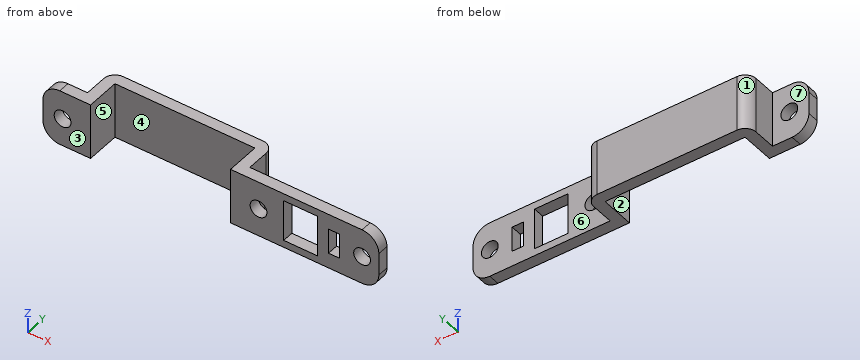
from build123d import *

# Parameters (mm, degrees)
EXTRUIR_L_MINA1_DEPTH = 10
CROQUIS2_R            = 1.5
CORTAR_EXTRUIR1_DEPTH = 61.141499815
REDONDEO2_R           = 3
REDONDEO3_R           = 2
CROQUIS3_W            = 6
CROQUIS3_H            = 7.4
CROQUIS3_W_2          = 2
CROQUIS3_H_2          = 4.5
CORTAR_EXTRUIR2_DEPTH = 61.141499815


with BuildPart() as part:
    # Croquis1 → Extruir-Lámina1 (new body)
    with BuildSketch(Plane.XY):
        Polygon((-1, 0), (0, 0), (7.5, 0), (7.5, 6), (32.5, 6), (32.5, 0), (41.5, 0), (59, 0), (59, 2), (41.5, 2), (34.5, 2), (34.5, 8), (5.5, 8), (5.5, 2), (0, 2), (-1, 2), align=None)
    extrude(amount=-EXTRUIR_L_MINA1_DEPTH)

    # Croquis2 → Cortar-Extruir1 (cut, through all)
    with BuildSketch(Plane(origin=(0, 2, 0), x_dir=(1, 0, 0), z_dir=(0, 1, 0))):
        with Locations(Location((2.5, 5, 0), (0, 0, 270))):
            Circle(CROQUIS2_R)
        with Locations(Location((37.5, 5, 0), (0, 0, 270))):
            Circle(CROQUIS2_R)
        with Locations(Location((56, 5, 0), (0, 0, 270))):
            Circle(CROQUIS2_R)
    extrude(amount=-CORTAR_EXTRUIR1_DEPTH, mode=Mode.SUBTRACT)

    # Redondeo2
    redondeo2_edges = [part.edges().sort_by_distance(p)[0] for p in [
        (-1, 1, 0),
        (59, 1, 0),
        (-1, 1, -10),
        (59, 1, -10),
    ]]
    fillet(redondeo2_edges, radius=REDONDEO2_R)

    # Redondeo3
    redondeo3_edges = [part.edges().sort_by_distance(p)[0] for p in [
        (5.5, 8, -5),
        (34.5, 8, -5),
    ]]
    fillet(redondeo3_edges, radius=REDONDEO3_R)

    # Croquis3 → Cortar-Extruir2 (cut, through all)
    with BuildSketch(Plane(origin=(0, 2, 0), x_dir=(1, 0, 0), z_dir=(0, 1, 0))):
        with Locations((45, 5)):
            Rectangle(CROQUIS3_W, CROQUIS3_H)
        with Locations((51, 5)):
            Rectangle(CROQUIS3_W_2, CROQUIS3_H_2)
    extrude(amount=-CORTAR_EXTRUIR2_DEPTH, mode=Mode.SUBTRACT)


solid = part.part
Source: CAD feature listing. Evaluate the final solid. Frame: model axes, mm. Face numbers are marked on the shaded views. A direction names the side the tool comes from. Round coordinates to 2 decimals unless told otherwise and drop trailing zeros. Loops run counter-clockwise (first coordinate to the right, second up) from the corner with the lowest first, then second, coordinate; pieces in that order, holes last. Notation, with made-up numbers: M 53,-19.75 L 63,-19.75 A18 cw 63,-13.75 Z; hole C 4,0.25 d5. An arc over 180 degrees is marked long. Return JSON: item names as keys, results as strings. Group by question number.
1. Pin query (flat end, axial travel): pin 1 (2.5 mm diameter, centred on x = 56, z = -5, fed in from +Y); pin 2 (1 mm diameter, centred on y = 2, z = -8.5, fed in from +X); pin 3 (5 mm diameter, centred on x = 24.5, z = -7.5, fed in from -Y); pin 4 (1 mm diameter, centred on x = 41.5, z = -6, fed in from +Y). Return the tip coordinate at first contact, or that it passes through.
2. Section query B-B on z = -5. State how many separate pieces and enclosed holes the cut face has, and give its area (3 significant figures).
3. Section query C-C on x = 37.5. Output: boundary loops of the cut face in (y, z), and give its area (3 significant figures).
4. Material intervals for line 1 along X through (y, z) = (1.5, -3.25); line 2 along X through (y, z) = (0.5, -2); line 3 along X through (y, z) = (4.5, -2.5), sorted ascending. Write a range as from..to.
5. Section query D-D on y = 4.5. Output: boundary loops of the cut face in (x, z), and give its area (3 significant figures).
6. Section query A-A on y = 1. Output: boundary loops of the cut face in (x, z), and give its area (3 significant figures).
7. Reachability of the marked faces 5, 6 and 7 from +Z, -Z, +X, -X, +Y, -Y: full face, straight path, thin tool, end or side. Return the list, or none.
8. Mould query, pull axis X, two halves, no side actions, for the marked faces 1, 2, 3 and 4. Classes: released by +X, released by -X, zero draft, split by the parting line, or undercut.
Checks:
{
 "1": {"pin 1": "passes through", "pin 2": "stops at x = 58.83", "pin 3": "stops at y = 6", "pin 4": "stops at y = 2"},
 "2": {"separate pieces": "6", "enclosed holes": "0", "area": "108 mm²"},
 "3": {"outline": "M 0,-10 L 2,-10 L 2,-6.5 L 0,-6.5 Z; M 0,-3.5 L 2,-3.5 L 2,0 L 0,0 Z", "area": "14.0 mm²"},
 "4": {"line 1": "x = -1..7.5, 32.5..42, 48..50, 52..59", "line 2": "x = -0.83..7.5, 32.5..42, 48..58.83", "line 3": "x = 5.5..7.5, 32.5..34.5"},
 "5": {"outline": "M 5.5,-10 L 7.5,-10 L 7.5,0 L 5.5,0 Z; M 32.5,-10 L 34.5,-10 L 34.5,0 L 32.5,0 Z", "area": "40.0 mm²"},
 "6": {"outline": "M -1,-7 A3 ccw 2,-10 L 7.5,-10 L 7.5,0 L 2,0 A3 ccw -1,-3 Z; M 32.5,-10 L 56,-10 A3 ccw 59,-7 L 59,-3 A3 ccw 56,0 L 32.5,0 Z; hole C 2.5,-5 d3; hole C 37.5,-5 d3; hole M 42,-8.7 L 48,-8.7 L 48,-1.3 L 42,-1.3 Z; hole M 50,-7.25 L 52,-7.25 L 52,-2.75 L 50,-2.75 Z; hole C 56,-5 d3", "area": "268 mm²"},
 "7": {"face 5": "+Z, -Z, -Y", "face 6": "+Z, -Z, +X, +Y", "face 7": "+Z, -Z, -X, +Y"},
 "8": {"face 1": "released by -X", "face 2": "undercut", "face 3": "zero draft", "face 4": "undercut"}
}
